Work out the finished part from the listing and answer in its coordinate system (mm). Face numbers are marked on the shaded views. A direction names the side the tool comes from. Round coordinates to 2 decimals unless told otherwise and drop trailing zeros. Order: outer loops, then holes, each group sorted by start corner. A loop starts at its lowest first (then second) coordinate and runs counter-clockwise, first axis right, second up. Notation, with made-up numbers: (25, 44) - (76, 44) arc R19 cw to (76, 48) - close; hole circle Ø1 at (-26, 47). An arc over 180 degrees is marked (long way). Put each result on its own line as item: value.
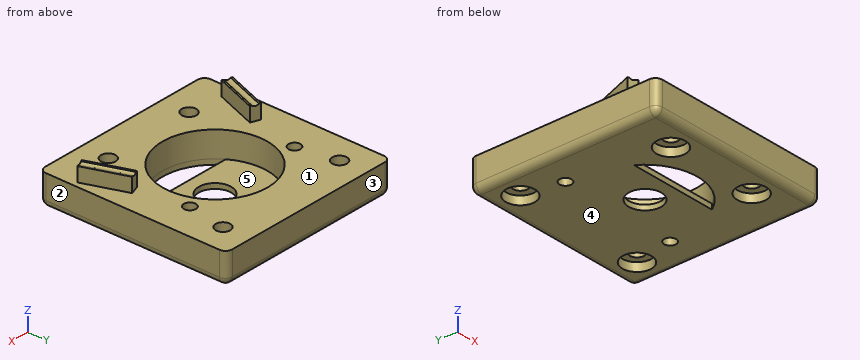
```python
from build123d import *

# Parameters (mm, degrees)
SKETCH1_W           = 55
SKETCH1_H           = 55
BOSS_EXTRUDE1_DEPTH = 9
SKETCH3_R           = 1.75
SKETCH3_R_2         = 2.15
CUT_EXTRUDE1_DEPTH  = 79.300702423
FILLET1_R           = 2
SKETCH4_R           = 4.25
CUT_EXTRUDE2_DEPTH  = 2.5
BOSS_EXTRUDE2_DEPTH = 13.027575483
BOSS_EXTRUDE3_DEPTH = 13.027575483
SKETCH7_R           = 15.392304845
CUT_EXTRUDE3_DEPTH  = 7.5
SKETCH8_R           = 4.75
CUT_EXTRUDE4_DEPTH  = 79.653460169
CUT_EXTRUDE5_DEPTH  = 79.653460169


with BuildPart() as part:
    # Sketch1 → Boss-Extrude1 (new body)
    with BuildSketch(Plane.XY):
        with Locations((27.5, 27.5)):
            Rectangle(SKETCH1_W, SKETCH1_H)
    extrude(amount=BOSS_EXTRUDE1_DEPTH)

    # Sketch3 → Cut-Extrude1 (cut, through all)
    with BuildSketch(Plane(origin=(0, 0, 0), x_dir=(-1, 0, 0), z_dir=(0, 0, -1))):
        with Locations((-45, 35.5)):
            Circle(SKETCH3_R)
        with Locations((-47, 47)):
            Circle(SKETCH3_R_2)
        with Locations((-8, 47)):
            Circle(SKETCH3_R_2)
        with Locations((-14, 8)):
            Circle(SKETCH3_R_2)
        with Locations((-41, 8)):
            Circle(SKETCH3_R_2)
        with Locations((-10, 35.5)):
            Circle(SKETCH3_R)
    extrude(amount=-CUT_EXTRUDE1_DEPTH, mode=Mode.SUBTRACT)

    # Fillet1
    fillet1_edges = [part.edges().sort_by_distance(p)[0] for p in [
        (27.5, 55, 0),
        (55, 27.5, 0),
        (27.5, 0, 0),
        (0, 27.5, 0),
        (0, 55, 4.5),
        (55, 55, 4.5),
        (55, 0, 4.5),
        (0, 0, 4.5),
    ]]
    fillet(fillet1_edges, radius=FILLET1_R)

    # Sketch4 → Cut-Extrude2 (cut)
    with BuildSketch(Plane(origin=(0, 0, 0), x_dir=(-1, 0, 0), z_dir=(0, 0, -1))):
        with Locations((-47, 47)):
            Circle(SKETCH4_R)
        with Locations((-8, 47)):
            Circle(SKETCH4_R)
        with Locations((-14, 8)):
            Circle(SKETCH4_R)
        with Locations((-41, 8)):
            Circle(SKETCH4_R)
    extrude(amount=-CUT_EXTRUDE2_DEPTH, mode=Mode.SUBTRACT)

    # Sketch5 → Boss-Extrude2 (add)
    with BuildSketch(Plane(origin=(3.091937938, -8.495029668, 0), x_dir=(0, 0, 1), z_dir=(-0.3420201433256653, 0.9396926207859098, 0))):
        with BuildLine():
            Line((13.177619471, 53.639405858), (9, 53.639405858))
            Line((9, 53.639405858), (9, 50.839405858))
            Line((9, 50.839405858), (13.177619471, 50.839405858))
            Line((13.177619471, 50.839405858), (13.177619471, 51.339405858))
            ThreePointArc((13.177619471, 51.339405858), (12.85, 52.239405858), (13.177619471, 53.139405858))
            Line((13.177619471, 53.139405858), (13.177619471, 53.639405858))
        make_face()
    extrude(amount=BOSS_EXTRUDE2_DEPTH)

    # Sketch6 → Boss-Extrude3 (add)
    with BuildSketch(Plane(origin=(3.341839876, 9.181629599, 0), x_dir=(0, 0, 1), z_dir=(-0.3420201433256654, -0.9396926207859095, 0))):
        with BuildLine():
            Line((13.177619471, 1.956311715), (9, 1.956311715))
            Line((9, 1.956311715), (9, -0.843688285))
            Line((9, -0.843688285), (13.177619471, -0.843688285))
            Line((13.177619471, -0.843688285), (13.177619471, -0.343688285))
            ThreePointArc((13.177619471, -0.343688285), (12.85, 0.556311715), (13.177619471, 1.456311715))
            Line((13.177619471, 1.456311715), (13.177619471, 1.956311715))
        make_face()
    extrude(amount=-BOSS_EXTRUDE3_DEPTH)

    # Sketch7 → Cut-Extrude3 (cut)
    with BuildSketch(Plane.XY.offset(9)):
        with Locations((27.5, 27.5)):
            Circle(SKETCH7_R)
    extrude(amount=-CUT_EXTRUDE3_DEPTH, mode=Mode.SUBTRACT)

    # Sketch8 → Cut-Extrude4 (cut, through all)
    with BuildSketch(Plane.XY.offset(1.5)):
        with Locations((27.5, 27.5)):
            Circle(SKETCH8_R)
    extrude(amount=-CUT_EXTRUDE4_DEPTH, mode=Mode.SUBTRACT)

    # Sketch10 → Cut-Extrude5 (cut, through all)
    with BuildSketch(Plane.XY.offset(1.5)):
        with BuildLine():
            Line((14.5, 19.258455942), (40.5, 19.258455942))
            ThreePointArc((40.5, 19.258455942), (27.5, 12.107695155), (14.5, 19.258455942))
        make_face()
    extrude(amount=-CUT_EXTRUDE5_DEPTH, mode=Mode.SUBTRACT)


solid = part.part
```
1) For a pull along X with two mould halves and no side action, classify the marked faces 1, 2 and 3 as pulls with the +X half, pulls with the -X half, needs draft (parallel to the pull), parting line crosses it, or undercut.
Findings below:
face 1: undercut
face 2: pulls with the +X half
face 3: needs draft
2) Given pin 1 Ø7 at (x, y) = (47, 47) entering from -Z; pin 2 Ø16.5 at (x, y) = (22, 38.5) entering from +Z; pin 3 Ø2 at (x, y) = (22.5, 34) entering from +Z, each flat-ended and moving along its own axis, determine where each tip first touches the part or whether it passes through.
Findings below:
pin 1: stops at z = 2.5
pin 2: stops at z = 9
pin 3: stops at z = 1.5
3) A cutting plane is placed at D-D on x = 44. Write down the section's boundary in (y, z), then the cut area to 3 significant figures.
Findings below:
outline: (0, 2) arc R2 ccw to (2, 0) - (4.99, 0) - (4.99, 2.5) - (11.01, 2.5) - (11.01, 0) - (34.06, 0) - (34.06, 9) - (0, 9) - close; (36.94, 0) - (43.99, 0) - (43.99, 2.5) - (50.01, 2.5) - (50.01, 0) - (53, 0) arc R2 ccw to (55, 2) - (55, 9) - (36.94, 9) - close
area: 437 mm2
4) A cutting plane is placed at B-B on y = 45.5. Write down the section's boundary in (x, z), then the cut area to 3 significant figures.
Findings below:
outline: (0, 2) arc R2 ccw to (2, 0) - (4.02, 0) - (4.02, 2.5) - (6.46, 2.5) - (6.46, 9) - (0, 9) - close; (9.54, 2.5) - (11.98, 2.5) - (11.98, 0) - (43.02, 0) - (43.02, 2.5) - (45.46, 2.5) - (45.46, 9) - (9.54, 9) - close; (48.54, 2.5) - (50.98, 2.5) - (50.98, 0) - (53, 0) arc R2 ccw to (55, 2) - (55, 9) - (48.54, 9) - close
area: 413 mm2
5) For the marked faces 4 and 5, determine the directions among +Z, -Z, +X, -X, +Y, -Y from which every point of the face is accessible in a straight line to the end or side of a thin tool.
Findings below:
face 4: -Z, +X, -X, +Y, -Y
face 5: +Z
6) Straight lines are drawn through the part: L1, parallel to Y at x = 41, z = 4.75; L2, parallel to Y at x = 27.5, z = 0.75; L3, parallel to Y at x = 27.5, z = 4.25. For each, find the intervals that lie inside material, in ascending order. Write a range as from..to.
Findings below:
L1: y = 0..5.85, 10.15..20.11, 34.89..55
L2: y = 0.44..12.11, 19.26..22.75, 32.25..54.56
L3: y = 0..12.11, 42.89..55
7) A cutting plane is placed at C-C on z = 11.25. Write down the section's boundary in (x, y), then the cut area to 3 significant figures.
Findings below:
outline: (1.5, 9.85) - (4.13, 8.89) - (8.59, 21.13) - (5.96, 22.09) - close; (46.41, 21.13) - (50.87, 8.89) - (53.5, 9.85) - (49.04, 22.09) - close
area: 73.0 mm2
8) A cutting plane is placed at A-A on z = 7. Write down the section's boundary in (x, y), then the cut area to 3 significant figures.
Findings below:
outline: (0, 2) arc R2 ccw to (2, 0) - (53, 0) arc R2 ccw to (55, 2) - (55, 53) arc R2 ccw to (53, 55) - (2, 55) arc R2 ccw to (0, 53) - close; hole circle Ø4.3 at (8, 47); hole circle Ø3.5 at (10, 35.5); hole circle Ø4.3 at (14, 8); hole circle Ø30.78 at (27.5, 27.5); hole circle Ø4.3 at (41, 8); hole circle Ø3.5 at (45, 35.5); hole circle Ø4.3 at (47, 47)
area: 2,200 mm2
